For this review, take the finished solid that the model builds, in its own axes (mm). Round coordinates to 2 decimals unless told otherwise and drop trailing zeros. Write each loop counter-clockwise with the first axis right and the second up, starting at its lowest first coordinate (ties: lowest second). Pieces come first, ordered by that corner, then holes.
from build123d import *

# Parameters (mm, degrees)
F0_W           = 127
F0_H           = 127
F1_DEPTH       = 3.175
F3_D           = 3.4544
F3_CSINK_D     = 3.556
F3_CSINK_ANGLE = 82
F4_D           = 3.4544
F4_CSINK_D     = 3.81
F4_CSINK_ANGLE = 82
F5_D           = 2.8448
F5_CSINK_D     = 3.048
F5_CSINK_ANGLE = 82
F6_D           = 3.2639


with BuildPart() as f1:
    # F0 (on Top) → F1 (new body)
    with BuildSketch(Plane.XY):
        Rectangle(F0_W, F0_H)
        with BuildLine():
            Line((-28.2575, 33.02), (28.2575, 33.02))
            ThreePointArc((28.2575, 33.02), (31.6250960454, 31.6250960454), (33.02, 28.2575))
            Line((33.02, 28.2575), (33.02, -28.2575))
            ThreePointArc((33.02, -28.2575), (31.6250960454, -31.6250960454), (28.2575, -33.02))
            Line((28.2575, -33.02), (-28.2575, -33.02))
            ThreePointArc((-28.2575, -33.02), (-31.6250960454, -31.6250960454), (-33.02, -28.2575))
            Line((-33.02, -28.2575), (-33.02, 28.2575))
            ThreePointArc((-33.02, 28.2575), (-31.6250960454, 31.6250960454), (-28.2575, 33.02))
        make_face(mode=Mode.SUBTRACT)
    extrude(amount=F1_DEPTH)

    # F3 (through all)
    with Locations(Plane.XY.offset(3.175)):
        with Locations((-53.34, 53.34), (53.34, 53.34), (53.34, -53.34), (-53.34, -53.34)):
            CounterSinkHole(F3_D / 2, F3_CSINK_D / 2, counter_sink_angle=F3_CSINK_ANGLE)

    # F4 (through all)
    with Locations(Plane.XY.offset(3.175)):
        with Locations((-25.4, 47.625), (0, 47.625), (25.4, 47.625), (-47.625, 25.4), (-47.625, 0), (-47.625, -25.4), (-25.4, -47.625), (0, -47.625), (25.4, -47.625), (47.625, -25.4), (47.625, 0), (47.625, 25.4)):
            CounterSinkHole(F4_D / 2, F4_CSINK_D / 2, counter_sink_angle=F4_CSINK_ANGLE)

    # F5 (through all)
    with Locations(Plane.XY.offset(3.175)):
        with Locations((-36.83, 19.05), (-36.83, -19.05), (36.83, 19.05), (36.83, -19.05)):
            CounterSinkHole(F5_D / 2, F5_CSINK_D / 2, counter_sink_angle=F5_CSINK_ANGLE)

    # F6 (through all)
    with Locations(Plane.XY.offset(3.175)):
        with Locations((-36.83, 0), (-19.05, 36.83), (0, 36.83), (19.05, 36.83), (36.83, 0), (19.05, -36.83), (0, -36.83), (-19.05, -36.83)):
            Hole(F6_D / 2)


solid = f1.part
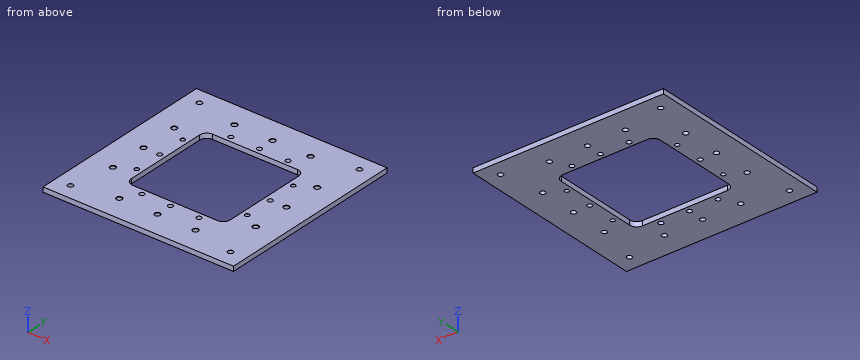
(1) We need section B-B, the plane x = 19.05. Give the boundary of the cut face in (y, z) (3 decimals).
Geometry check:
outline: (-63.5, 0) - (-38.462, 0) - (-38.462, 3.175) - (-63.5, 3.175) - close; (-35.198, 0) - (-33.02, 0) - (-33.02, 3.175) - (-35.198, 3.175) - close; (33.02, 0) - (35.198, 0) - (35.198, 3.175) - (33.02, 3.175) - close; (38.462, 0) - (63.5, 0) - (63.5, 3.175) - (38.462, 3.175) - close
(2) We need section D-D, the plane x = -15.5. Give the boundary of the cut face in (y, z) (3 decimals).
Geometry check:
outline: (-63.5, 0) - (-33.02, 0) - (-33.02, 3.175) - (-63.5, 3.175) - close; (33.02, 0) - (63.5, 0) - (63.5, 3.175) - (33.02, 3.175) - close
(3) For line 1 along Y through (x, z) = (-25.4, 0.85); line 2 along X through (y, z) = (-19.05, 1.5); line 3 along Y through (x, z) = (-19.05, 0.65), list the stretches that pass through material, from the lowest coordinate up.
Geometry check:
line 1: y = -63.5 to -49.35, -45.9 to -33.02, 33.02 to 45.9, 49.35 to 63.5
line 2: x = -63.5 to -38.25, -35.41 to -33.02, 33.02 to 35.41, 38.25 to 63.5
line 3: y = -63.5 to -38.46, -35.2 to -33.02, 33.02 to 35.2, 38.46 to 63.5
(4) We need section C-C, the plane y = 0. Give the boundary of the cut face in (x, z) (3 decimals).
Geometry check:
outline: (-63.5, 0) - (-49.352, 0) - (-49.352, 2.97) - (-49.53, 3.175) - (-63.5, 3.175) - close; (-45.898, 0) - (-38.462, 0) - (-38.462, 3.175) - (-45.72, 3.175) - (-45.898, 2.97) - close; (-35.198, 0) - (-33.02, 0) - (-33.02, 3.175) - (-35.198, 3.175) - close; (33.02, 0) - (35.198, 0) - (35.198, 3.175) - (33.02, 3.175) - close; (38.462, 0) - (45.898, 0) - (45.898, 2.97) - (45.72, 3.175) - (38.462, 3.175) - close; (49.352, 0) - (63.5, 0) - (63.5, 3.175) - (49.53, 3.175) - (49.352, 2.97) - close
(5) We need section A-A, the plane y = 25.4. Give the boundary of the cut face in (x, z) (3 decimals).
Geometry check:
outline: (-63.5, 0) - (-49.352, 0) - (-49.352, 2.97) - (-49.53, 3.175) - (-63.5, 3.175) - close; (-45.898, 0) - (-33.02, 0) - (-33.02, 3.175) - (-45.72, 3.175) - (-45.898, 2.97) - close; (33.02, 0) - (45.898, 0) - (45.898, 2.97) - (45.72, 3.175) - (33.02, 3.175) - close; (49.352, 0) - (63.5, 0) - (63.5, 3.175) - (49.53, 3.175) - (49.352, 2.97) - close
